The model under review builds one solid part; all positions refer to its coordinate system, in mm. Face numbers are marked on the shaded views. Give positions to 0.01 mm unless a question says otherwise; leave off trailing zeros. Loops run counter-clockwise (first coordinate to the right, second up) from the corner with the lowest first, then second, coordinate; pieces in that order, holes last. Notation, with made-up numbers: M 44,69 L 61,69 A20 ccw 61,85 Z; hole C 35,57.25 d4. An arc over 180 degrees is marked long. Put each result on its own line as item: value. Start each with the question number.
from build123d import *

# Parameters (mm, degrees)
SKETCH1_R      = 8
SKETCH1_R_2    = 5
EXTRUDE1_DEPTH = 15
SKETCH2_R      = 16
SKETCH2_R_2    = 5
SKETCH2_R_3    = 1.9
EXTRUDE2_DEPTH = 4


with BuildPart() as part:
    # Sketch1 → Extrude1 (new body)
    with BuildSketch(Plane.XY):
        Circle(SKETCH1_R)
        Circle(SKETCH1_R_2, mode=Mode.SUBTRACT)
    extrude(amount=EXTRUDE1_DEPTH)

    # Sketch2 → Extrude2 (add)
    with BuildSketch(Plane.XY.offset(15)):
        Circle(SKETCH2_R)
        Circle(SKETCH2_R_2, mode=Mode.SUBTRACT)
        with Locations((-8.485281374, 8.485281374)):
            Circle(SKETCH2_R_3, mode=Mode.SUBTRACT)
        with Locations((8.485281374, 8.485281374)):
            Circle(SKETCH2_R_3, mode=Mode.SUBTRACT)
        with Locations((-8.485281374, -8.485281374)):
            Circle(SKETCH2_R_3, mode=Mode.SUBTRACT)
        with Locations((8.485281374, -8.485281374)):
            Circle(SKETCH2_R_3, mode=Mode.SUBTRACT)
    extrude(amount=EXTRUDE2_DEPTH)


solid = part.part
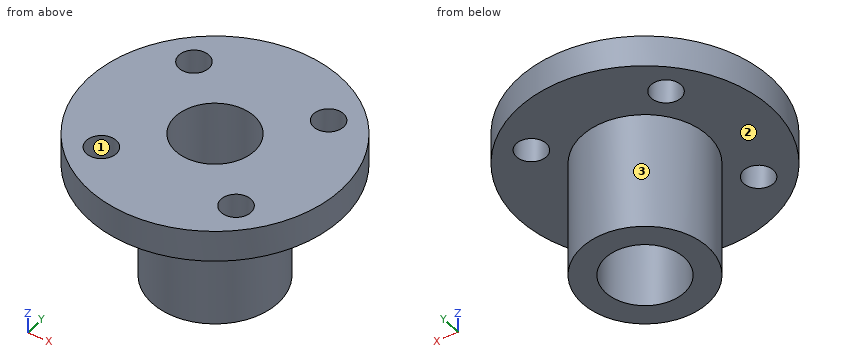
(1) To check wall thickness, follow L1, parallel to Y at x = -10, z = 17.75; L2, parallel to Y at x = 0, z = 6.25; L3, parallel to Z at x = -14, y = -4. State the ranges of each line that lie inside material, in increasing order. Write a range as [from, to].
(2) We need section D-D, the plane y = -5.5. Write out the cut boundary in (x, z), plus the area to 3 significant figures.
(3) Draft analysis for pull direction Y (two halves, no side actions). For the marked faces 1, 2 and 3, state which applies: +Y half, -Y half, draft (parallel to the pull), parting line (faces both ways), or undercut.
(4) We need section C-C, the plane z = 12.5. Write out the cut boundary in (x, y), plus the area to 3 significant figures.
(5) We need section A-A, the plane y = 0. Write out the cut boundary in (x, z).
(6) Insertion check: pin 1 (4.5 mm diameter, centred on x = 8.49, y = -8.49, fed in from -Z); pin 2 (4 mm diameter, centred on x = -8, z = 6.5, fed in from +Y); pin 3 (10 mm diameter, centred on y = -3, z = 9, fed in from +X). Each pin has a flat end and moves straight along its axis. Give the tip position at first contact, or say it passes through.
Check sheet entries:
1. L1: y = [-12.49, -9.63], [-7.34, 7.34], [9.63, 12.49]
1. L2: y = [-8, -5], [5, 8]
1. L3: z = [15, 19]
2. outline: M -15.02,15 L -5.81,15 L -5.81,0 L 5.81,0 L 5.81,15 L 15.02,15 L 15.02,19 L -15.02,19 Z
2. area: 294 mm²
3. face 1: undercut
3. face 2: draft
3. face 3: parting line
4. outline: C 0,0 d16; hole C 0,0 d10
4. area: 123 mm²
5. outline: M -16,15 L -8,15 L -8,0 L -5,0 L -5,19 L -16,19 Z; M 5,0 L 8,0 L 8,15 L 16,15 L 16,19 L 5,19 Z
6. pin 1: stops at z = 15
6. pin 2: stops at y = 5.29
6. pin 3: stops at x = 8
